from build123d import *

# Parameters (mm, degrees)
SKETCH1_W                      = 38
SKETCH1_H                      = 38
BOSS_EXTRUDE1_DEPTH            = 15
SKETCH2_R                      = 16
CUT_EXTRUDE1_DEPTH             = 10
SKETCH2_3_R                    = 14
CUT_EXTRUDE3_DEPTH             = 31.773365107
FILLET1_R                      = 4
CBORE_FOR_M2_SHCS1_D           = 2.6
CBORE_FOR_M2_SHCS1_CBORE_D     = 4.4
CBORE_FOR_M2_SHCS1_CBORE_DEPTH = 2
CUT_EXTRUDE4_DEPTH             = 2
BOSS_EXTRUDE3_DEPTH            = 5


with BuildPart() as part:
    # Sketch1 → Boss-Extrude1 (new body)
    with BuildSketch(Plane(origin=(0, 0, 0), x_dir=(1, 0, 0), z_dir=(0, 1, 0))):
        Rectangle(SKETCH1_W, SKETCH1_H)
    extrude(amount=BOSS_EXTRUDE1_DEPTH)

    # Sketch2 → Cut-Extrude1 (cut)
    with BuildSketch(Plane(origin=(0, 15, 0), x_dir=(1, 0, 0), z_dir=(0, 1, 0))):
        with Locations(Location((0, 0, 0), (0, 0, 270))):
            Circle(SKETCH2_R)
    extrude(amount=-CUT_EXTRUDE1_DEPTH, mode=Mode.SUBTRACT)

    # Sketch2_3 → Cut-Extrude3 (cut, through all)
    with BuildSketch(Plane(origin=(0, 15, 0), x_dir=(1, 0, 0), z_dir=(0, 1, 0))):
        with Locations(Location((0, 0, 0), (0, 0, 270))):
            Circle(SKETCH2_3_R)
    extrude(amount=-CUT_EXTRUDE3_DEPTH, mode=Mode.SUBTRACT)

    # Fillet1
    fillet1_edges = [part.edges().sort_by_distance(p)[0] for p in [
        (19, 7.5, 19),
        (-19, 7.5, 19),
        (-19, 7.5, -19),
        (19, 7.5, -19),
    ]]
    fillet(fillet1_edges, radius=FILLET1_R)

    # CBORE for M2 SHCS1 (through all)
    with Locations(Plane(origin=(0, 15, 0), x_dir=(1, 0, 0), z_dir=(0, 1, 0))):
        with Locations((-15, 15), (15, 15), (-15, -15), (15, -15)):
            CounterBoreHole(CBORE_FOR_M2_SHCS1_D / 2, CBORE_FOR_M2_SHCS1_CBORE_D / 2, CBORE_FOR_M2_SHCS1_CBORE_DEPTH)

    # Sketch6 → Cut-Extrude4 (cut)
    with BuildSketch(Plane.XZ):
        Polygon((0.343583705, 2.476277496), (0.481017187, 3.466788495), (19, -15.155263686), (19, -16.283973067), align=None)
    extrude(amount=-CUT_EXTRUDE4_DEPTH, mode=Mode.SUBTRACT)

    # Sketch7 → Boss-Extrude3 (add)
    with BuildSketch(Plane(origin=(0, 15, 0), x_dir=(1, 0, 0), z_dir=(0, 1, 0))):
        Polygon((-19, 11.221825407), (-16.171572875, 8.393398282), (-19, 5.564971157), align=None)
        Polygon((11.932562755, 19), (10.700479231, 15.194481614), (15, 19), align=None)
    extrude(amount=BOSS_EXTRUDE3_DEPTH)


solid = part.part
Can you work these out from the model? Positions are in its coordinate system, mm. A direction names the side the tool comes from. Coordinates: 2 decimals unless noted, no trailing zeros. Write each loop counter-clockwise with the first axis right and the second up, starting at its lowest first coordinate (ties: lowest second). Pieces come first, ordered by that corner, then holes. Notation, with made-up numbers: (-32.75, -28.5) -> (22.25, -28.5) arc R31 ccw to (22.25, 9.5) -> close; hole circle Ø2 at (-12, -25). An arc over 180 degrees is marked (long way). Answer as CSV lines item,"result".
1) If we mould it in two halves opening along Z, with no side actions, what happens to faces 1 (the cylindrical face through (-12.968, 14.014, 15.843)), 2 (the cylindrical face through (17.797, 7.605, 17.859)), 3 (the flat face through (-13, 0, 8))? For each: +Z half, -Z half, draft (parallel to the pull), parting line (faces both ways), or undercut.
Check result:
face 1,"undercut"
face 2,"+Z half"
face 3,"draft"
2) Will these pins go through, and if not, where does the flat tip stop? P1, Ø5, axis at x = 9, z = 9, coming from the -Y side; P2, Ø2, axis at x = 16, z = 14.5, coming from the +Y side; P3, Ø3.5, axis at x = 16, z = -15.5, coming from the +Y side.
Check result:
P1,"y = 0"
P2,"y = 13"
P3,"y = 15"
3) If I drill on line 1 (X direction, y = 4.5, z = -15); line 2 (X direction, y = 6.25, z = 0.5), over which ranges is the centre line in solid material (lowest first)? Write a range as from..to.
Check result:
line 1,"-19..-16.3, -13.7..13.7, 16.3..19"
line 2,"-19..-15.99, 15.99..19"
4) If we section it at C-C on z = 0: Please give me the cut outline in (x, y).
Check result:
outline,"(-19, 0) -> (-14, 0) -> (-14, 5) -> (-16, 5) -> (-16, 15) -> (-19, 15) -> close; (14, 0) -> (19, 0) -> (19, 15) -> (16, 15) -> (16, 5) -> (14, 5) -> close"
5) If we section it at B-B on y = 11.5: Please give me the cut outline in (x, z), then the cut area to 3 significant figures.
Check result:
outline,"(-19, -15) arc R4 ccw to (-15, -19) -> (15, -19) arc R4 ccw to (19, -15) -> (19, 15) arc R4 ccw to (15, 19) -> (-15, 19) arc R4 ccw to (-19, 15) -> close; hole circle Ø2.6 at (-15, -15); hole circle Ø2.6 at (-15, 15); hole circle Ø32 at (0, 0); hole circle Ø2.6 at (15, -15); hole circle Ø2.6 at (15, 15)"
area,"605 mm²"
6) If we section it at A-A on x = 0: Please give me the cut outline in (y, z), then the cut area to 3 significant figures.
Check result:
outline,"(0, -19) -> (15, -19) -> (15, -16) -> (5, -16) -> (5, -14) -> (0, -14) -> close; (0, 14) -> (5, 14) -> (5, 16) -> (15, 16) -> (15, 19) -> (0, 19) -> close"
area,"110 mm²"
7) If we section it at D-D on x = 14.5: Count the separate pieces of the cut face and the enclosed holes in it, then the cut area to 3 significant figures.
Check result:
separate pieces,"3"
enclosed holes,"0"
area,"355 mm²"
8) On a 3-axis mill with a long thin cutter (end or side, diameter ignored), from which of +Z, -Z, +X, -X, +Y, -Y can I reach the whole of each face in a straight line? I mean faces 4 (the flat face through (-17.566, 17.465, -6.999)), 5 (the flat face through (15, 2, -12)), 6 (the flat face through (-17.61, 17.46, -9.83)). Say none if no direction works.
Check result:
face 4,"+Z, +X, +Y"
face 5,"-Y"
face 6,"-Z, +X, +Y"
